```python
from build123d import *

# Parameters (mm, degrees)
F0_W          = 58.8
F0_H          = 80.5
F1_DEPTH      = 6.5
F2_W          = 52.8
F2_H          = 74.5
F3_DEPTH      = 3.5
F5_R          = 3.5
F6_DEPTH      = 3.5
F8_R          = 1.45
F10_R         = 1.45
F11_DEPTH     = 6.501
F9_R          = 1.6
F7_R          = 1.6
F12_DEPTH     = 1.6
F13_W         = 36.8
F13_H         = 3
F14_DEPTH     = 3.5
F15_W         = 24.6
F15_H         = 3
F16_DEPTH     = 5.5
F19_DEPTH     = 2.2
F20_R         = 1
F21_DEPTH     = 6.501
F22_T1_DEPTH  = 11
F22_T3_DEPTH  = 52.8
F22_T5_DEPTH  = 74.5
F22_S9_W      = 3
F22_S9_H      = 3
F22_T10_DEPTH = 3
F22_S15_W     = 3
F22_S15_H     = 3
F22_T16_DEPTH = 3
F22_S21_W     = 3
F22_S21_H     = 3
F22_T22_DEPTH = 3
F22_S27_W     = 3
F22_S27_H     = 3
F22_T28_DEPTH = 3
F24_R         = 2
F25_R         = 1.5
F26_R         = 2
F27_R         = 2.75
F28_DEPTH     = 1.6


# Not quite as in the source:
# - a fillet or chamfer that OpenCascade refuses, or shapes differently, is made with other operations: its cross-section is extruded or revolved along the edge and cut away or added
# - a feature of the source that left no trace in its solid (it failed there, or was rolled back) is left out


with BuildPart() as f1:
    # F0 (on Top) → F1 (new body)
    with BuildSketch(Plane.XY):
        with Locations((29.4, 40.25)):
            Rectangle(F0_W, F0_H)
    extrude(amount=F1_DEPTH)

    # F2 (on face) → F3 (cut)
    with BuildSketch(Plane.XY.offset(6.5)):
        with Locations((29.4, 40.25)):
            Rectangle(F2_W, F2_H)
    extrude(amount=-F3_DEPTH, mode=Mode.SUBTRACT)

    # F5 (on face) → F6 (join)
    with BuildSketch(Plane.XY.offset(3)):
        with Locations((7.75, 7.375)):
            Circle(F5_R)
        with Locations((7.75, 73.125)):
            Circle(F5_R)
        with Locations((51.05, 73.125)):
            Circle(F5_R)
        with Locations((51.05, 7.375)):
            Circle(F5_R)
    extrude(amount=F6_DEPTH)

    # F8 (on face) + F10 (on face) → F11 (cut, through all)
    with BuildSketch(Plane.XY.offset(6.5)):
        with Locations((51.05, 73.125)):
            Circle(F8_R)
    with BuildSketch(Plane.XY.offset(6.5)):
        with Locations((7.75, 7.375)):
            Circle(F10_R)
    extrude(amount=-F11_DEPTH, mode=Mode.SUBTRACT)

    # F9 (on face) + F7 (on face) → F12 (cut)
    with BuildSketch(Plane.XY.offset(6.5)):
        with Locations((7.75, 73.125)):
            Circle(F9_R)
    with BuildSketch(Plane.XY.offset(6.5)):
        with Locations((51.05, 7.375)):
            Circle(F7_R)
    extrude(amount=-F12_DEPTH, mode=Mode.SUBTRACT)

    # F13 (on face) → F14 (cut)
    with BuildSketch(Plane.XY.offset(6.5)):
        with Locations((29.4, 79)):
            Rectangle(F13_W, F13_H)
    extrude(amount=-F14_DEPTH, mode=Mode.SUBTRACT)

    # F15 (on face) → F16 (cut)
    with BuildSketch(Plane.XY.offset(6.5)):
        with Locations((25.5, 1.5)):
            Rectangle(F15_W, F15_H)
    extrude(amount=-F16_DEPTH, mode=Mode.SUBTRACT)

    # F17 (on face) + F18 (on face) → F19 (cut)
    with BuildSketch(Plane.XY.offset(6.5)):
        Polygon((47.8, 79), (47.8, 77.5), (55.8, 77.5), (55.8, 3), (37.8, 3), (37.8, 1.5), (57.3, 1.5), (57.3, 79), align=None)
    with BuildSketch(Plane.XY.offset(6.5)):
        Polygon((1.5, 1.5), (13.2, 1.5), (13.2, 3), (3, 3), (3, 77.5), (11, 77.5), (11, 79), (1.5, 79), align=None)
    extrude(amount=-F19_DEPTH, mode=Mode.SUBTRACT)

    # F20 (on face) → F21 (cut, through all)
    with BuildSketch(Plane(origin=(0, 0, 0), x_dir=(1, 0, 0), z_dir=(0, 0, -1))):
        with Locations((39.3, -5)):
            Circle(F20_R)
        with Locations((38.3, -75.5)):
            Circle(F20_R)
        with Locations((24.55, -75.5)):
            Circle(F20_R)
    extrude(amount=-F21_DEPTH, mode=Mode.SUBTRACT)

    # F22: fillet of radius 3 on 8 edges, made by hand

    # F22_s2 → F22_t1 (cut)
    with BuildSketch(Plane.XY.offset(3)):
        with BuildLine():
            ThreePointArc((0, 3), (0.8786796564, 0.8786796564), (3, 0))
            Line((3, 0), (0, 0))
            Line((0, 0), (0, 3))
        make_face()
        with BuildLine():
            ThreePointArc((55.8, 0), (57.9213203436, 0.8786796564), (58.8, 3))
            Line((58.8, 3), (58.8, 0))
            Line((58.8, 0), (55.8, 0))
        make_face()
        with BuildLine():
            ThreePointArc((0, 77.5), (0.8786796564, 79.6213203436), (3, 80.5))
            Line((3, 80.5), (0, 80.5))
            Line((0, 80.5), (0, 77.5))
        make_face()
        with BuildLine():
            ThreePointArc((55.8, 80.5), (57.9213203436, 79.6213203436), (58.8, 77.5))
            Line((58.8, 77.5), (58.8, 80.5))
            Line((58.8, 80.5), (55.8, 80.5))
        make_face()
    extrude(amount=F22_T1_DEPTH, mode=Mode.SUBTRACT)

    # F22_s4 → F22_t3 (cut)
    with BuildSketch(Plane.YZ.offset(3)):
        with BuildLine():
            ThreePointArc((0, 3), (0.8786796564, 0.8786796564), (3, 0))
            Line((3, 0), (0, 0))
            Line((0, 0), (0, 3))
        make_face()
        with BuildLine():
            ThreePointArc((80.5, 3), (79.6213203436, 0.8786796564), (77.5, 0))
            Line((77.5, 0), (80.5, 0))
            Line((80.5, 0), (80.5, 3))
        make_face()
    extrude(amount=F22_T3_DEPTH, mode=Mode.SUBTRACT)

    # F22_s6 → F22_t5 (cut)
    with BuildSketch(Plane.XZ.offset(-77.5)):
        with BuildLine():
            ThreePointArc((0, 3), (0.8786796564, 0.8786796564), (3, 0))
            Line((3, 0), (0, 0))
            Line((0, 0), (0, 3))
        make_face()
        with BuildLine():
            ThreePointArc((55.8, 0), (57.9213203436, 0.8786796564), (58.8, 3))
            Line((58.8, 3), (58.8, 0))
            Line((58.8, 0), (55.8, 0))
        make_face()
    extrude(amount=F22_T5_DEPTH, mode=Mode.SUBTRACT)


with BuildPart() as f22_tool8:
    # F22_s9 → F22_t10 (new body)
    with BuildSketch(Plane.YZ.offset(3)):
        with Locations((1.5, 1.5)):
            Rectangle(F22_S9_W, F22_S9_H)
    extrude(amount=-F22_T10_DEPTH)

    # F22_s11 → F22_t12 (revolve, cut)
    with BuildSketch(Plane(origin=(3, 3, 3), x_dir=(0, 0.7071067812, 0.7071067812), z_dir=(0, -0.7071067812, 0.7071067812))):
        with BuildLine():
            ThreePointArc((0, -3), (3, 0), (0, 3))
            Line((0, 3), (0, -3))
        make_face()
    revolve(axis=Axis((3, 3, 3), (-1, 0, 0)), mode=Mode.SUBTRACT)


with BuildPart() as f1_1:
    add(f1.part)

    # F22_t7: cut F22_tool8
    add(f22_tool8.part, mode=Mode.SUBTRACT)


with BuildPart() as f22_tool14:
    # F22_s15 → F22_t16 (new body)
    with BuildSketch(Plane.YZ.offset(55.8)):
        with Locations((1.5, 1.5)):
            Rectangle(F22_S15_W, F22_S15_H)
    extrude(amount=F22_T16_DEPTH)

    # F22_s17 → F22_t18 (revolve, cut)
    with BuildSketch(Plane(origin=(55.8, 3, 3), x_dir=(0, 0.7071067812, 0.7071067812), z_dir=(0, 0.7071067812, -0.7071067812))):
        with BuildLine():
            ThreePointArc((0, -3), (3, 0), (0, 3))
            Line((0, 3), (0, -3))
        make_face()
    revolve(axis=Axis((55.8, 3, 3), (1, 0, 0)), mode=Mode.SUBTRACT)


with BuildPart() as f1_2:
    add(f1_1.part)

    # F22_t13: cut F22_tool14
    add(f22_tool14.part, mode=Mode.SUBTRACT)


with BuildPart() as f22_tool20:
    # F22_s21 → F22_t22 (new body)
    with BuildSketch(Plane.YZ.offset(3)):
        with Locations((79, 1.5)):
            Rectangle(F22_S21_W, F22_S21_H)
    extrude(amount=-F22_T22_DEPTH)

    # F22_s23 → F22_t24 (revolve, cut)
    with BuildSketch(Plane(origin=(3, 77.5, 3), x_dir=(0, -0.7071067812, 0.7071067812), z_dir=(0, -0.7071067812, -0.7071067812))):
        with BuildLine():
            ThreePointArc((0, -3), (3, 0), (0, 3))
            Line((0, 3), (0, -3))
        make_face()
    revolve(axis=Axis((3, 77.5, 3), (-1, 0, 0)), mode=Mode.SUBTRACT)


with BuildPart() as f1_3:
    add(f1_2.part)

    # F22_t19: cut F22_tool20
    add(f22_tool20.part, mode=Mode.SUBTRACT)


with BuildPart() as f22_tool26:
    # F22_s27 → F22_t28 (new body)
    with BuildSketch(Plane.XZ.offset(-77.5)):
        with Locations((57.3, 1.5)):
            Rectangle(F22_S27_W, F22_S27_H)
    extrude(amount=-F22_T28_DEPTH)

    # F22_s29 → F22_t30 (revolve, cut)
    with BuildSketch(Plane(origin=(55.8, 77.5, 3), x_dir=(-0.7071067812, 0, 0.7071067812), z_dir=(-0.7071067812, 0, -0.7071067812))):
        with BuildLine():
            ThreePointArc((0, -3), (3, 0), (0, 3))
            Line((0, 3), (0, -3))
        make_face()
    revolve(axis=Axis((55.8, 77.5, 3), (0, 1, 0)), mode=Mode.SUBTRACT)


with BuildPart() as f1_4:
    add(f1_3.part)

    # F22_t25: cut F22_tool26
    add(f22_tool26.part, mode=Mode.SUBTRACT)

    # F24
    f24_edges = [f1_4.edges().sort_by_distance(p)[0] for p in [
        (57.3, 79, 5.4),
        (57.3, 1.5, 5.4),
        (1.5, 1.5, 5.4),
        (1.5, 79, 5.4),
    ]]
    fillet(f24_edges, radius=F24_R)

    # F25#2 (call 1 of 2: OpenCascade refuses the feature's edges together)
    f25_2_edges = [f1_4.edges().sort_by_distance(p)[0] for p in [
        (47.8, 79, 3),
    ]]
    fillet(f25_2_edges, radius=F25_R)

    # F25 (call 2 of 2)
    f25_edges = [f1_4.edges().sort_by_distance(p)[0] for p in [
        (11, 79, 3),
    ]]
    fillet(f25_edges, radius=F25_R)

    # F26
    f26_edges = [f1_4.edges().sort_by_distance(p)[0] for p in [
        (13.2, 1.881966, 1),
        (37.8, 1.881966, 1),
    ]]
    fillet(f26_edges, radius=F26_R)

    # F27 (on face) → F28 (cut)
    with BuildSketch(Plane(origin=(0, 0, 0), x_dir=(1, 0, 0), z_dir=(0, 0, -1))):
        with Locations((51.05, -73.125)):
            Circle(F27_R)
        with Locations((7.75, -7.375)):
            Circle(F27_R)
    extrude(amount=-F28_DEPTH, mode=Mode.SUBTRACT)


solid = f1_4.part
```
Geometry: final body of the model. Coordinates: model frame, mm. A direction names the side the tool comes from. Round coordinates to 2 decimals unless told otherwise and drop trailing zeros. Write each loop counter-clockwise with the first axis right and the second up, starting at its lowest first coordinate (ties: lowest second). Pieces come first, ordered by that corner, then holes. Notation, with made-up numbers: M -19.5,8 L -15.5,8 A18 ccw -15.5,35 Z; hole C 57,57.25 d4. An arc over 180 degrees is marked long. Answer in a Markdown table with one row per item. Add a question column.
(1) Draft query along Y for faces 5 (the face through (48.27, 71, 4.73)), 6 (the face through (0.86, 40.77, 0.9)), 7 (the face through (51.788, 5.956, 5.711)), 8 (the face through (51, 80.5, 5)). Return one class per face: pulls with the +Y half, pulls with the -Y half, needs draft (parallel to the pull), parting line crosses it, or undercut.
(2) Contact query for flat-ended pins moving along their axis: pin 1 (6 mm diameter, centred on x = 19.5, y = 57.5, fed in from +Z); pin 2 (1 mm diameter, centred on x = 51, y = 7.5, fed in from +Z); pin 3 (12 mm diameter, centred on x = 6, y = 17.5, fed in from +Z); pin 4 (0.8 mm diameter, centred on y = 80, z = 5.5, fed in from +X). Output: stop coordinate, or through.
(3) Cut plane B-B, the plane y = 48. Return the cut outline in (x, z).
(4) Ray query, L1, parallel to Y at x = 7.75, z = 3.05 (3 decimals); L2, parallel to Y at x = 7.75, z = 4.6 (3 decimals); L3, parallel to Y at x = 55.5, z = 5.25. Return the intervals inside material, ascending.
(5) Cut plane D-D, the plane x = 24.55. Return the cut outline in (y, z).
(6) Cut plane C-C, the plane x = 30.5. Return the cut outline in (y, z).
(7) Reachability of faces 1 (the face through (11.45, 79.02, 3.43)), 2 (the face through (1.5, 41, 5)), 3 (the face through (10.3, 8.4, 0.8)), 4 (the face through (51.72, 71.84, 4.08)) from +Z, -Z, +X, -X, +Y, -Y: full face, straight path, thin tool, end or side. Return the list, or none.
Established:
| question | item | result |
|---|---|---|
| 1 | face 5 | undercut |
| 1 | face 6 | needs draft |
| 1 | face 7 | undercut |
| 1 | face 8 | pulls with the +Y half |
| 2 | pin 1 | z = 3 |
| 2 | pin 2 | z = 4.9 |
| 2 | pin 3 | z = 6.5 |
| 2 | pin 4 | x = 57.94 |
| 3 | outline | M 0,3 A3 ccw 3,0 L 55.8,0 A3 ccw 58.8,3 L 58.8,6.5 L 57.3,6.5 L 57.3,4.3 L 55.8,4.3 L 55.8,3 L 3,3 L 3,4.3 L 1.5,4.3 L 1.5,6.5 L 0,6.5 Z |
| 4 | L1 | 0 to 3, 3.875 to 5.925, 8.825 to 10.875, 69.625 to 76.625, 77.5 to 80.5 |
| 4 | L2 | 0 to 1.5, 3.875 to 5.925, 8.825 to 10.875, 69.625 to 76.625, 79 to 80.5 |
| 4 | L3 | 0 to 1.51, 78.99 to 80.5 |
| 5 | outline | M 0.76,1 A3 ccw 3,0 L 74.5,0 L 74.5,3 L 3,3 L 3,1 Z; M 76.5,0 L 77.5,0 A3 ccw 80.5,3 L 76.5,3 Z |
| 6 | outline | M 0.76,1 A3 ccw 3,0 L 77.5,0 A3 ccw 80.5,3 L 3,3 L 3,1 Z |
| 7 | face 1 | +Z, +Y |
| 7 | face 2 | +Z |
| 7 | face 3 | -Z |
| 7 | face 4 | +Z, -Z |
